```python
from build123d import *

# Parameters (mm, degrees)
SKETCH3_W           = 67.056
SKETCH3_H           = 35.13836
BOSS_EXTRUDE1_DEPTH = 3.175
SKETCH4_W           = 9.579428572
SKETCH4_H           = 3.175
BOSS_EXTRUDE3_DEPTH = 3.175
LPATTERN1_COUNT     = 3
LPATTERN1_PITCH     = 19.158857143


with BuildPart() as part:
    # Sketch3 → Boss-Extrude1 (new body)
    with BuildSketch(Plane.XY):
        with Locations((-33.528, 17.56918)):
            Rectangle(SKETCH3_W, SKETCH3_H)
    extrude(amount=BOSS_EXTRUDE1_DEPTH)

    # Sketch4 → Boss-Extrude3 (add)
    with BuildSketch(Plane.XY.offset(3.175)):
        with Locations((-52.686857143, -1.5875)):
            Rectangle(SKETCH4_W, SKETCH4_H)
    boss_extrude3 = extrude(amount=-BOSS_EXTRUDE3_DEPTH)

    # LPattern1: Boss-Extrude3 ×3
    with Locations(*[(i * LPATTERN1_PITCH, 0, 0) for i in range(1, LPATTERN1_COUNT)]):
        add(boss_extrude3)


solid = part.part
```
Here's how the part is built. I have some questions about the finished solid (model axes, mm). A direction names the side the tool comes from. Round coordinates to 2 decimals unless told otherwise and drop trailing zeros. Write each loop counter-clockwise with the first axis right and the second up, starting at its lowest first coordinate (ties: lowest second). Pieces come first, ordered by that corner, then holes.
Q1. Will these pins go through, and if not, where does the flat tip stop? P1, Ø1, axis at y = -1.5, z = 2, coming from the +X side; P2, Ø1, axis at x = -41.5, z = 2, coming from the -Y side.
Q2. If we mould it in two halves opening along X, with no side actions, what happens to faces 1 (the flat face through (0, 17, 2)), 2 (the flat face through (-14, -3.175, 2)), 3 (the flat face through (-43, 0, 2))? For each: +X half, -X half, draft (parallel to the pull), parting line (faces both ways), or undercut.
Q3. Please list where these lines run through material, in increasing order: probe 1 along X at (y, z) = (-0.5, 0.9); probe 2 along Y at (x, z) = (-19.5, 1.7).
Q4. Which directions (+Z, -Z, +X, -X, +Y, -Y) give clear straight access to the entire face, cutting with the end or side of a thin tool? Please do faces 4 (the flat face through (-24, 0, 2)), 5 (the flat face through (-9.579, -2, 2)), 6 (the flat face through (-57.477, -2, 2)), 7 (the flat face through (-34, 16, 0)).
Q5. If we section it at A-A on z = 2.15: Write out the boundary of the cut face in (x, y) (3 decimals).
Q6. If we section it at B-B on x = -27: Write out the boundary of the cut face in (y, z) (3 decimals), plus the area to 3 significant figures.
Answer below:
1. P1: stops at x = -9.58
1. P2: stops at y = 0
2. face 1: +X half
2. face 2: draft
2. face 3: undercut
3. probe 1: x = -57.48 to -47.9, -38.32 to -28.74, -19.16 to -9.58
3. probe 2: y = 0 to 35.14
4. face 4: +Z, -Z, -Y
4. face 5: +Z, -Z, +X, -Y
4. face 6: +Z, -Z, -X, -Y
4. face 7: -Z, +X, -X, +Y, -Y
5. outline: (-67.056, 0) - (-57.477, 0) - (-57.477, -3.175) - (-47.897, -3.175) - (-47.897, 0) - (-38.318, 0) - (-38.318, -3.175) - (-28.738, -3.175) - (-28.738, 0) - (-19.159, 0) - (-19.159, -3.175) - (-9.579, -3.175) - (-9.579, 0) - (0, 0) - (0, 35.138) - (-67.056, 35.138) - close
6. outline: (0, 0) - (35.138, 0) - (35.138, 3.175) - (0, 3.175) - close
6. area: 112 mm2
